from build123d import *

# Parameters (mm, degrees)
F1_DEPTH = 1.5
F3_DEPTH = 15
F5_DEPTH = 1.5
F7_DEPTH = 29
F8_DEPTH = 29


with BuildPart() as f1:
    # F0 (on Top) → F1 (new body)
    with BuildSketch(Plane.XY):
        with BuildLine():
            ThreePointArc((41.5, 33.5), (40.3284271247, 36.3284271247), (37.5, 37.5))
            Line((37.5, 37.5), (-37.5, 37.5))
            ThreePointArc((-37.5, 37.5), (-40.3284271247, 36.3284271247), (-41.5, 33.5))
            Line((-41.5, 33.5), (-41.5, -33.5))
            ThreePointArc((-41.5, -33.5), (-40.3284271247, -36.3284271247), (-37.5, -37.5))
            Line((-37.5, -37.5), (37.5, -37.5))
            ThreePointArc((37.5, -37.5), (40.3284271247, -36.3284271247), (41.5, -33.5))
            Line((41.5, -33.5), (41.5, 33.5))
        make_face()
    extrude(amount=F1_DEPTH)

    # F2 (on face) → F3 (join)
    with BuildSketch(Plane.XY.offset(1.5)):
        with BuildLine():
            Line((41.5, -33.5), (41.5, 33.5))
            ThreePointArc((41.5, 33.5), (40.3284271247, 36.3284271247), (37.5, 37.5))
            Line((37.5, 37.5), (-37.5, 37.5))
            ThreePointArc((-37.5, 37.5), (-40.3284271247, 36.3284271247), (-41.5, 33.5))
            Line((-41.5, 33.5), (-41.5, -33.5))
            ThreePointArc((-41.5, -33.5), (-40.3284271247, -36.3284271247), (-37.5, -37.5))
            Line((-37.5, -37.5), (37.5, -37.5))
            ThreePointArc((37.5, -37.5), (40.3284271247, -36.3284271247), (41.5, -33.5))
        make_face()
        with BuildLine():
            Line((-36, 36), (36, 36))
            ThreePointArc((36, 36), (38.8284271247, 34.8284271247), (40, 32))
            Line((40, 32), (40, -32))
            ThreePointArc((40, -32), (38.8284271247, -34.8284271247), (36, -36))
            Line((36, -36), (-36, -36))
            ThreePointArc((-36, -36), (-38.8284271247, -34.8284271247), (-40, -32))
            Line((-40, -32), (-40, 32))
            ThreePointArc((-40, 32), (-38.8284271247, 34.8284271247), (-36, 36))
        make_face(mode=Mode.SUBTRACT)
    extrude(amount=F3_DEPTH)

    # F4 (on face) → F5 (join)
    with BuildSketch(Plane.XY.offset(16.5)):
        with BuildLine():
            Line((45.5, -32), (45.5, -27.5))
            Line((45.5, -27.5), (66.5, -27.5))
            Line((66.5, -27.5), (66.5, 57.5))
            Line((66.5, 57.5), (-30.5, 57.5))
            Line((-30.5, 57.5), (-30.5, 41.5))
            Line((-30.5, 41.5), (-36, 41.5))
            ThreePointArc((-36, 41.5), (-42.0648066734, 38.373774392), (-44.5, 32))
            Line((-44.5, 32), (-44.5, -33.5))
            ThreePointArc((-44.5, -33.5), (-41.9782906023, -39.336308765), (-36, -41.5))
            Line((-36, -41.5), (36, -41.5))
            ThreePointArc((36, -41.5), (42.7175144213, -38.7175144213), (45.5, -32))
        make_face()
        with BuildLine():
            Line((41.5, 33.5), (41.5, -33.5))
            ThreePointArc((41.5, -33.5), (40.3284271247, -36.3284271247), (37.5, -37.5))
            Line((37.5, -37.5), (-37.5, -37.5))
            ThreePointArc((-37.5, -37.5), (-40.3284271247, -36.3284271247), (-41.5, -33.5))
            Line((-41.5, -33.5), (-41.5, 33.5))
            ThreePointArc((-41.5, 33.5), (-40.3284271247, 36.3284271247), (-37.5, 37.5))
            Line((-37.5, 37.5), (37.5, 37.5))
            ThreePointArc((37.5, 37.5), (40.3284271247, 36.3284271247), (41.5, 33.5))
        make_face(mode=Mode.SUBTRACT)
        with BuildLine():
            ThreePointArc((37.5, -37.5), (40.3284271247, -36.3284271247), (41.5, -33.5))
            Line((41.5, -33.5), (41.5, 33.5))
            ThreePointArc((41.5, 33.5), (40.3284271247, 36.3284271247), (37.5, 37.5))
            Line((37.5, 37.5), (-37.5, 37.5))
            ThreePointArc((-37.5, 37.5), (-40.3284271247, 36.3284271247), (-41.5, 33.5))
            Line((-41.5, 33.5), (-41.5, -33.5))
            ThreePointArc((-41.5, -33.5), (-40.3284271247, -36.3284271247), (-37.5, -37.5))
            Line((-37.5, -37.5), (37.5, -37.5))
        make_face()
        with BuildLine():
            ThreePointArc((-40, 32), (-38.8284271247, 34.8284271247), (-36, 36))
            Line((-36, 36), (36, 36))
            ThreePointArc((36, 36), (38.8284271247, 34.8284271247), (40, 32))
            Line((40, 32), (40, -32))
            ThreePointArc((40, -32), (38.8284271247, -34.8284271247), (36, -36))
            Line((36, -36), (-36, -36))
            ThreePointArc((-36, -36), (-38.8284271247, -34.8284271247), (-40, -32))
            Line((-40, -32), (-40, 32))
        make_face(mode=Mode.SUBTRACT)
    extrude(amount=F5_DEPTH)

    # F6 (on face) → F7 (join)
    with BuildSketch(Plane.XY.offset(18)):
        Polygon((-36, 41.5), (-36, 39.5), (-28.5, 39.5), (-28.5, 55.5), (64.5, 55.5), (64.5, -25.5), (43.5, -25.5), (43.5, -32), (45.5, -32), (45.5, -27.5), (66.5, -27.5), (66.5, 57.5), (-30.5, 57.5), (-30.5, 41.5), align=None)
    extrude(amount=F7_DEPTH)

    # F6 (on face) → F8 (join)
    with BuildSketch(Plane.XY.offset(18)):
        with BuildLine():
            ThreePointArc((-42.5, 32), (-40.6488749734, 36.9623583103), (-36, 39.5))
            Line((-36, 39.5), (-36, 41.5))
            ThreePointArc((-36, 41.5), (-42.0648066734, 38.373774392), (-44.5, 32))
            Line((-44.5, 32), (-44.5, -33.5))
            ThreePointArc((-44.5, -33.5), (-41.9782906023, -39.336308765), (-36, -41.5))
            Line((-36, -41.5), (36, -41.5))
            ThreePointArc((36, -41.5), (42.7175144213, -38.7175144213), (45.5, -32))
            Line((45.5, -32), (43.5, -32))
            ThreePointArc((43.5, -32), (41.3033008589, -37.3033008589), (36, -39.5))
            Line((36, -39.5), (-36, -39.5))
            ThreePointArc((-36, -39.5), (-40.4229515032, -37.7706974618), (-42.5, -33.5))
            Line((-42.5, -33.5), (-42.5, 32))
        make_face()
    extrude(amount=F8_DEPTH)


solid = f1.part
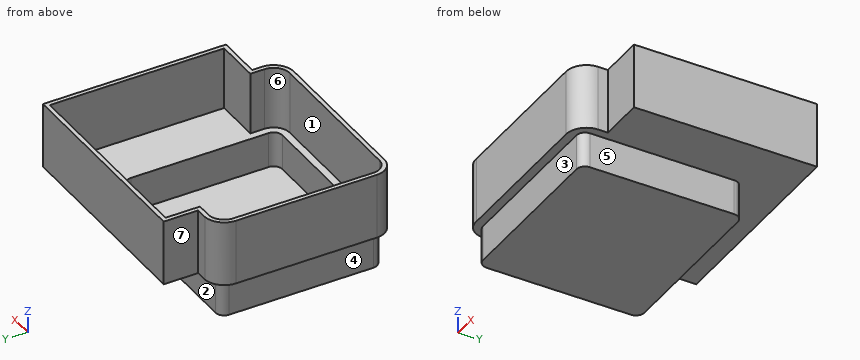
For this review, take the finished solid that the model builds, in its own axes (mm). Face numbers are marked on the shaded views. A direction names the side the tool comes from. Give positions to 0.01 mm unless a question says otherwise; leave off trailing zeros. Loops run counter-clockwise (first coordinate to the right, second up) from the corner with the lowest first, then second, coordinate; pieces in that order, holes last. Notation, with made-up numbers: M -30.75,15.5 L 27.25,15.5 A22 ccw 27.25,54.5 Z; hole C 5,19 d6. An arc over 180 degrees is marked long. Answer as a JSON object with one key per item and string values. Group by question number.
Q1. Mouldability with a two-part tool opening along X and no side actions: class the marked faces 5, 6 and 7 as +X half, -X half, draft (parallel to the pull), parting line (faces both ways), or undercut.
Q2. Add section C-C on x = -7. Give the boundary of the cut face in (y, z).
Q3. Tool access review of the marked faces 1, 2, 3 and 4: name each direction out of +Z, -Z, +X, -X, +Y, -Y from which nothing blocks a thin tool from reaching the whole face with its end or side.
Q4. Add section A-A on z = 38.5. Give the boundary of the cut face in (x, y), and give its area (3 significant figures).
Q5. Add section B-B on y = 12.5. Give the boundary of the cut face in (x, z), and give its area (3 significant figures).
Q6. For probe 1 along X at (y, z) = (-12, 15); probe 2 along X at (y, z) = (-20, 24); probe 3 along Y at (x, z) = (-2, 34), list the stretches that pass through material, from the lowest coordinate up. Write a range as [from, to].
Q7. Insertion check: P1, Ø17, axis at x = 59, z = 25, coming from the -Y side; P2, Ø8, axis at y = -13.5, z = 12, coming from the -X side; P3, Ø2, axis at x = -31.5, z = 39, coming from the -Y side. Each pin has a flat end and moves straight along its axis. Give the tip position at first contact, or say it passes through.
Q8. Add section D-D on z = 8. Give the boundary of the cut face in (x, y), and give its area (3 significant figures).
Checked values:
{
 "1": {"face 5": "+X half", "face 6": "undercut", "face 7": "-X half"},
 "2": {"outline": "M -41.5,16.5 L -37.5,16.5 L -37.5,0 L 37.5,0 L 37.5,16.5 L 57.5,16.5 L 57.5,47 L 55.5,47 L 55.5,18 L 36,18 L 36,1.5 L -36,1.5 L -36,18 L -39.5,18 L -39.5,47 L -41.5,47 Z"},
 "3": {"face 1": "+Z", "face 2": "-Z, +X, -X, +Y", "face 3": "-Z, +X, -X, -Y", "face 4": "-Z, -X, +Y, -Y"},
 "4": {"outline": "M -44.5,-33.5 A8.01 ccw -36,-41.5 L 36,-41.5 A9.5 ccw 45.5,-32 L 45.5,-27.5 L 66.5,-27.5 L 66.5,57.5 L -30.5,57.5 L -30.5,41.5 L -36,41.5 A9.56 ccw -44.5,32 Z; hole M -42.5,-33.5 A6.52 ccw -36,-39.5 L 36,-39.5 A7.5 ccw 43.5,-32 L 43.5,-25.5 L 64.5,-25.5 L 64.5,55.5 L -28.5,55.5 L -28.5,39.5 L -36,39.5 A7.58 ccw -42.5,32 Z", "area": "805 mm²"},
 "5": {"outline": "M -44.5,16.5 L -41.5,16.5 L -41.5,0 L 41.5,0 L 41.5,16.5 L 66.5,16.5 L 66.5,47 L 64.5,47 L 64.5,18 L 40,18 L 40,1.5 L -40,1.5 L -40,18 L -42.5,18 L -42.5,47 L -44.5,47 Z", "area": "332 mm²"},
 "6": {"probe 1": "[-41.5, -40], [40, 41.5]", "probe 2": "[-44.5, -42.5], [64.5, 66.5]", "probe 3": "[-41.5, -39.5], [55.5, 57.5]"},
 "7": {"P1": "y = -27.5", "P2": "x = -41.5", "P3": "y = -41.5"},
 "8": {"outline": "M -41.5,-33.5 A4 ccw -37.5,-37.5 L 37.5,-37.5 A4 ccw 41.5,-33.5 L 41.5,33.5 A4 ccw 37.5,37.5 L -37.5,37.5 A4 ccw -41.5,33.5 Z; hole M -40,-32 A4 ccw -36,-36 L 36,-36 A4 ccw 40,-32 L 40,32 A4 ccw 36,36 L -36,36 A4 ccw -40,32 Z", "area": "465 mm²"}
}
